The model under review builds one solid part; all positions refer to its coordinate system, in mm. A direction names the side the tool comes from. Round coordinates to 2 decimals unless told otherwise and drop trailing zeros. Write each loop counter-clockwise with the first axis right and the second up, starting at its lowest first coordinate (ties: lowest second). Pieces come first, ordered by that corner, then holes. Notation, with made-up numbers: (-7, 85.5) -> (47, 85.5) arc R17 ccw to (47, 89.5) -> close; hole circle Ø10 at (66, 64.5). An arc over 180 degrees is marked (long way). Answer as a JSON object with one key per item and string values. Group by question number.
1) To check wall thickness, follow probe 1 along X at (y, z) = (-0.75, 6.75); probe 2 along X at (y, z) = (8.35, 4.5); probe 3 along Y at (x, z) = (6.5, 1.5). State the ranges of each line that lie inside material, in increasing order. Write a range as [from, to].
2) We need section B-B, the plane z = 4.5. Write out the cut boundary in (x, y).
3) Machinability: for faces 1 (the cylindrical face through (16.62, 8.88, 8.14)), 2 (the flat face through (11, 7.646, 4)), 3 (the cylindrical face through (0.92, 9.29, 4.56)), 4 (the flat face through (-53, 7.646, 4)), which of the approach directions +Z, -Z, +X, -X, +Y, -Y give a long, thin tool a straight path to every point of the face, cutting with its end or side? Answer none if there is none.
4) Insertion check: pin 1 Ø8 at (x, y) = (-33, -7.5) entering from -Z (3 decimals); pin 2 Ø2 at (y, z) = (-1, 5.5) entering from -X; pin 3 Ø4.5 at (y, z) = (-8, 3) entering from +X; pin 4 Ø1.8 at (x, z) = (12.52, 4.5) entering from -Y. Each pin has a flat end and moves straight along its axis. Give the tip position at first contact, or say it passes through.
5) We need section C-C, the plane x = -7. Write out the cut boundary in (y, z).
6) Mouldability with a two-part tool opening along X and no side actions: class faces 5 (the cylindrical face through (-59.578, 8.913, 0.855)), 6 (the flat face through (-42.981, -3, 4)), 7 (the flat face through (10, 10.146, 4)), 8 (the cylindrical face through (11.738, 8.913, 4.327)) as pulls with the +X half, pulls with the -X half, needs draft (parallel to the pull), parting line crosses it, or undercut.
7) We need section A-A, the plane y = -3. Write out the cut boundary in (x, z), then the cut area to 3 significant figures.
from build123d import *

# Parameters (mm, degrees)
BOSS_EXTRUDE1_DEPTH = 9
SKETCH2_R           = 0.8
CUT_EXTRUDE1_DEPTH  = 9
FILLET1_R           = 1
FILLET2_R           = 3
FILLET3_R           = 3


with BuildPart() as part:
    # Sketch1 → Boss-Extrude1 (new body)
    with BuildSketch(Plane.XY):
        Polygon((-45.480536292, -17.354415164), (-45.480536292, 7.645584836), (-60.480536292, 7.645584836), (-60.480536292, 10.145584836), (-42.980536292, 10.145584836), (-42.980536292, -14.854415164), (0.019463708, -14.854415164), (0.019463708, 10.145584836), (17.519463708, 10.145584836), (17.519463708, 7.645584836), (2.519463708, 7.645584836), (2.519463708, -17.354415164), align=None)
    extrude(amount=BOSS_EXTRUDE1_DEPTH)

    # Sketch2 → Cut-Extrude1 (cut)
    with BuildSketch(Plane(origin=(0, 10.145584836, 0), x_dir=(1, 0, 0), z_dir=(0, 1, 0))):
        with Locations(Location((-55.480536292, -4.5, 0), (0, 0, 270))):
            Circle(SKETCH2_R)
        with Locations(Location((12.519463708, -4.5, 0), (0, 0, 270))):
            Circle(SKETCH2_R)
    extrude(amount=-CUT_EXTRUDE1_DEPTH, mode=Mode.SUBTRACT)

    # Fillet1
    fillet1_edges = [part.edges().sort_by_distance(p)[0] for p in [
        (-45.480536292, 7.645584836, 4.5),
        (-42.980536292, -14.854415164, 4.5),
        (0.019463708, -14.854415164, 4.5),
        (2.519463708, 7.645584836, 4.5),
    ]]
    fillet(fillet1_edges, radius=FILLET1_R)

    # Fillet2
    fillet2_edges = [part.edges().sort_by_distance(p)[0] for p in [
        (-45.480536292, -17.354415164, 4.5),
        (-42.980536292, 10.145584836, 4.5),
        (0.019463708, 10.145584836, 4.5),
        (2.519463708, -17.354415164, 4.5),
    ]]
    fillet(fillet2_edges, radius=FILLET2_R)

    # Fillet3
    fillet3_edges = [part.edges().sort_by_distance(p)[0] for p in [
        (-60.480536292, 8.895584836, 0),
        (17.519463708, 8.895584836, 0),
        (17.519463708, 8.895584836, 9),
        (-60.480536292, 8.895584836, 9),
    ]]
    fillet(fillet3_edges, radius=FILLET3_R)


solid = part.part
Here are the results:
{
 "1": {"probe 1": "x = [-45.48, -42.98], [0.02, 2.52]", "probe 2": "x = [-60.48, -56.28], [-54.68, -43.23], [0.27, 11.72], [13.32, 17.52]", "probe 3": "y = [7.65, 10.15]"},
 "2": {"outline": "(-60.48, 7.65) -> (-56.28, 7.65) -> (-56.28, 10.15) -> (-60.48, 10.15) -> close; (-54.68, 7.65) -> (-46.48, 7.65) arc R1 cw to (-45.48, 6.65) -> (-45.48, -14.35) arc R3 ccw to (-42.48, -17.35) -> (-0.48, -17.35) arc R3 ccw to (2.52, -14.35) -> (2.52, 6.65) arc R1 cw to (3.52, 7.65) -> (11.72, 7.65) -> (11.72, 10.15) -> (3.02, 10.15) arc R3 ccw to (0.02, 7.15) -> (0.02, -13.85) arc R1 cw to (-0.98, -14.85) -> (-41.98, -14.85) arc R1 cw to (-42.98, -13.85) -> (-42.98, 7.15) arc R3 ccw to (-45.98, 10.15) -> (-54.68, 10.15) -> close; (13.32, 7.65) -> (17.52, 7.65) -> (17.52, 10.15) -> (13.32, 10.15) -> close"},
 "3": {"face 1": "+Z, +X, +Y, -Y", "face 2": "+Z, -Z, +X, -Y", "face 3": "+Z, -Z, +Y", "face 4": "+Z, -Z, -X, -Y"},
 "4": {"pin 1": "passes through", "pin 2": "stops at x = -45.48", "pin 3": "stops at x = 2.52", "pin 4": "stops at y = 7.65"},
 "5": {"outline": "(-17.35, 0) -> (-14.85, 0) -> (-14.85, 9) -> (-17.35, 9) -> close"},
 "6": {"face 5": "pulls with the -X half", "face 6": "undercut", "face 7": "needs draft", "face 8": "undercut"},
 "7": {"outline": "(-45.48, 0) -> (-42.98, 0) -> (-42.98, 9) -> (-45.48, 9) -> close; (0.02, 0) -> (2.52, 0) -> (2.52, 9) -> (0.02, 9) -> close", "area": "45.0 mm^2"}
}
